CAD build for the part. Positions are in the model's coordinates, mm. Face numbers are marked on the shaded views. A direction names the side the tool comes from. Round coordinates to 2 decimals unless told otherwise and drop trailing zeros. Write each loop counter-clockwise with the first axis right and the second up, starting at its lowest first coordinate (ties: lowest second). Pieces come first, ordered by that corner, then holes. Notation, with made-up numbers: (-33, 75.5) - (0, 75.5) arc R21 ccw to (0, 107.5) - close; hole circle Ø1 at (-2, -34). An arc over 180 degrees is marked (long way). Put each result on its own line as item: value. Start each with the question number.
Item 1: Mould opens along Z. For the marked faces 4, 5, 6 and 7 say: released by +Z, released by -Z, zero draft, split by the parting line, or undercut.
Item 2: Drill centre lines: line 1 (Z direction, x = 93.25, y = 2); line 2 (X direction, y = 2, z = 2); line 3 (Z direction, x = 91.75, y = 6.75). Where is each one in solid material? Low to high. Write a range as from..to.
Item 3: Pin check, flat tips, straight feed: pin 1 Ø5 at (x, z) = (89, 29) entering from +Y; pin 2 Ø8 at (x, z) = (91, 32.5) entering from -Y. Stop position of each tip, or through.
Item 4: Cut at C-C (y = 9.5). Give the cut face in (x, z).
Item 5: 3-axis set-ups, long thin cutter, end or side, ignore diameter. For the marked faces 1, 2 and 3: which of +Z, -Z, +X, -X, +Y, -Y reach the whole face in a straight line?
Item 6: Cut at D-D (z = 34). Give the cut face in (x, y).
Item 7: Cut at A-A (z = 70.5). Give the cut face in (x, y).
Item 8: Cut at B-B (x = 88.5). Give the cut face in (y, z), and give its area (3 significant figures).
Autodesk Fusion 360 part; units mm, degrees
sketch "Sketch1" plane through (0, 0, 0) normal (0, 1, 0) x (1, 0, 0)
  line L0 (0, 0) -> (20.4, 0) construction
  line L1 (20.4, 0) -> (20.4, -88.85) construction
  line L2 (0, 0) -> (20.4, 0)
  line L3 (20.4, 0) -> (20.4, -88.85)
  line L4 (20.4, -88.85) -> (0, -88.85)
  line L5 (0, -88.85) -> (0, 0)
  line L6 (20.4, 0) -> (17.9, 0) construction
  line L7 (17.9, 0) -> (17.9, -2.5) construction
  line L8 (17.9, -2.5) -> (20.4, -2.5) construction
  line L9 (20.4, -2.5) -> (20.4, 0) construction
  circle A0 centre (17.9, -2.5) radius 1.5
  line L10 (0, 0) -> (2.5, 0) construction
  line L11 (2.5, 0) -> (2.5, -2.5) construction
  line L12 (2.5, -2.5) -> (0, -2.5) construction
  line L13 (0, -2.5) -> (0, 0) construction
  line L14 (0, -88.85) -> (2.5, -88.85) construction
  line L15 (2.5, -88.85) -> (2.5, -86.35) construction
  line L16 (2.5, -86.35) -> (0, -86.35) construction
  line L17 (0, -86.35) -> (0, -88.85) construction
  line L18 (20.4, -88.85) -> (17.9, -88.85) construction
  line L19 (17.9, -88.85) -> (17.9, -86.35) construction
  line L20 (17.9, -86.35) -> (20.4, -86.35) construction
  line L21 (20.4, -86.35) -> (20.4, -88.85) construction
  circle A1 centre (2.5, -86.35) radius 1.5
  circle A2 centre (17.9, -86.35) radius 1.5
  circle A3 centre (2.5, -2.5) radius 1.5
  circle A4 centre (2.5, -2.5) radius 2
  circle A5 centre (17.9, -2.5) radius 2
  circle A6 centre (2.5, -86.35) radius 2
  circle A7 centre (17.9, -86.35) radius 2
  dimension "d1" = 20.4
  dimension "d2" = 88.85
  dimension "d3" = 2.5
  dimension "d4" = 2.5
  dimension "d5" = 3
  dimension "d6" = 2.5
  dimension "d7" = 2.5
  dimension "d8" = 2.5
  dimension "d9" = 2.5
  dimension "d10" = 2.5
  dimension "d11" = 2.5
  dimension "d12" = 3
  dimension "d13" = 3
  dimension "d14" = 3
  dimension "d15" = 4
  dimension "d16" = 4
  dimension "d17" = 4
  dimension "d18" = 4
extrude "Extrude1" add sketch "Sketch1" along normal blind 1 contours L2 L3 L4 L5 makes body 1
extrude "Extrude2" add sketch "Sketch1" along normal blind 1 contours A0 | A1 | A2 | A3 | A4 | A5 | A6 | A7 bodies 1
extrude "Extrude3" add sketch "Sketch1" along normal blind 10 contours A4 | A5 | A6 | A7 bodies 1
extrude "Extrude4" add 4 faces at (17.7887, 1, 3.5508) (2.9404, 1, 2.5827) (17.4222, 1, 86.4974) (2.3887, 1, 87.4008) along direction (0, 1, 0) blind 5 on bodies 1 bodies 1
sketch "Sketch2" plane through (0, 0, 0) normal (0, 1, 0) x (1, 0, 0)
  line L0 (55, 0) -> (64.5, 0) construction
  line L1 (55, 0) -> (55, -75.2) construction
  line L2 (55, -75.2) -> (64.5, -75.2)
  line L3 (64.5, -75.2) -> (64.5, 0)
  line L4 (64.5, 0) -> (55, 0)
  line L5 (55, 0) -> (55, -75.2)
  line L6 (64.5, -75.2) -> (68.5, -75.2) construction
  line L7 (68.5, -75.2) -> (68.5, -79.2) construction
  line L8 (68.5, -79.2) -> (64.5, -79.2) construction
  line L9 (64.5, -79.2) -> (64.5, -75.2) construction
  line L10 (55, 0) -> (51, 0) construction
  line L11 (51, 0) -> (51, 4) construction
  line L12 (51, 4) -> (55, 4) construction
  line L13 (55, 4) -> (55, 0) construction
  line L14 (51, 4) -> (68.5, 4)
  line L15 (68.5, 4) -> (68.5, -79.2)
  line L16 (68.5, -79.2) -> (51, -79.2)
  line L17 (51, -79.2) -> (51, 4)
  line L18 (59.75, -75.2) -> (59.75, -61.2) construction
  line L19 (59.75, 0) -> (59.75, -14) construction
  line L20 (59.75, -14) -> (55, -14) construction
  line L21 (59.75, -61.2) -> (64.5, -61.2) construction
  line L22 (55, -14) -> (64.5, -14)
  line L23 (64.5, -14) -> (64.5, -61.2)
  line L24 (64.5, -61.2) -> (55, -61.2)
  line L25 (55, -61.2) -> (55, -14)
  line L26 (55, -75.2) -> (64.5, -75.2)
  line L27 (64.5, -75.2) -> (64.5, -79.2)
  line L28 (64.5, -79.2) -> (55, -79.2)
  line L29 (55, -79.2) -> (55, -75.2)
  line L30 (55, 0) -> (64.5, 0)
  line L31 (64.5, 0) -> (64.5, 4)
  line L32 (64.5, 4) -> (55, 4)
  line L33 (55, 4) -> (55, 0)
  dimension "d27" = 9.5
  dimension "d28" = 75.2
  dimension "d29" = 4
  dimension "d30" = 4
  dimension "d31" = 4
  dimension "d32" = 4
  dimension "d35" = 14
  dimension "d36" = 14
extrude "Extrude5" add sketch "Sketch2" along normal blind 1 separate body makes body 2
extrude "Extrude6" add sketch "Sketch2" along normal blind 10 contours L3 L5 L22 L23 L24 L25 bodies 2
extrude "Extrude7" add sketch "Sketch2" along normal blind 20 contours L5 L14 L16 L17 L25 L29 L33 | L3 L14 L15 L16 L23 L27 L31 bodies 2
sketch "Sketch3" plane through (0, 0, 0) normal (0, 1, 0) x (1, 0, 0)
  line L0 (85, -15) -> (94.5, -15)
  line L1 (94.5, -15) -> (94.5, -62.2)
  line L2 (94.5, -62.2) -> (85, -62.2)
  line L3 (85, -62.2) -> (85, -15)
  line L4 (94.5, -15) -> (96.5, -15)
  line L5 (96.5, -15) -> (96.5, -62.2)
  line L6 (96.5, -62.2) -> (94.5, -62.2)
  line L7 (94.5, -62.2) -> (94.5, -15)
  line L8 (85, -15) -> (83, -15)
  line L9 (83, -15) -> (83, -62.2)
  line L10 (83, -62.2) -> (85, -62.2)
  line L11 (85, -62.2) -> (85, -15)
  line L12 (85, -38.6) -> (85, -0.9) construction
  line L13 (94.5, -38.6) -> (94.5, -0.9) construction
  line L14 (85, -38.6) -> (85, -76.3) construction
  line L15 (94.5, -38.6) -> (94.5, -76.3) construction
  line L16 (83, -62.2) -> (85, -62.2)
  line L17 (85, -62.2) -> (85, -76.3)
  line L18 (85, -76.3) -> (83, -76.3)
  line L19 (83, -76.3) -> (83, -62.2)
  line L20 (94.5, -76.3) -> (96.5, -76.3)
  line L21 (96.5, -76.3) -> (96.5, -62.2)
  line L22 (96.5, -62.2) -> (94.5, -62.2)
  line L23 (94.5, -62.2) -> (94.5, -76.3)
  line L24 (83, -76.3) -> (96.5, -76.3)
  line L25 (96.5, -76.3) -> (96.5, -78.3)
  line L26 (96.5, -78.3) -> (83, -78.3)
  line L27 (83, -78.3) -> (83, -76.3)
  line L28 (85, -0.9) -> (83, -0.9)
  line L29 (83, -0.9) -> (83, -15)
  line L30 (83, -15) -> (85, -15)
  line L31 (85, -15) -> (85, -0.9)
  line L32 (94.5, -0.9) -> (96.5, -0.9)
  line L33 (96.5, -0.9) -> (96.5, -15)
  line L34 (96.5, -15) -> (94.5, -15)
  line L35 (94.5, -15) -> (94.5, -0.9)
  line L36 (96.5, -0.9) -> (83, -0.9)
  line L37 (83, -0.9) -> (83, 1.1)
  line L38 (83, 1.1) -> (96.5, 1.1)
  line L39 (96.5, 1.1) -> (96.5, -0.9)
  dimension "d41" = 9.5
  dimension "d42" = 47.2
  dimension "d43" = 2
  dimension "d44" = 2
  dimension "d49" = 37.7
  dimension "d50" = 37.7
  dimension "d51" = 37.7
  dimension "d52" = 37.7
  dimension "d53" = 2
  dimension "d54" = 2
extrude "Extrude8" add sketch "Sketch3" along normal blind 3 separate body contours L0 L1 L2 L3 L7 L11 makes body 3
extrude "Extrude9" add sketch "Sketch3" along normal blind 11 contours L3 L8 L9 L10 L11 L16 L30 | L1 L4 L5 L6 L7 L22 L34 bodies 3
extrude "Extrude10" add sketch "Sketch3" along normal blind 11 contours L8 L28 L29 L30 L31 L36 | L4 L32 L33 L34 L35 L36 | L10 L16 L17 L18 L19 L24 | L28 L32 L36 L37 L38 L39 | L6 L20 L21 L22 L23 L24 | L18 L20 L24 L25 L26 L27 bodies 3
hidden bodies 1 2
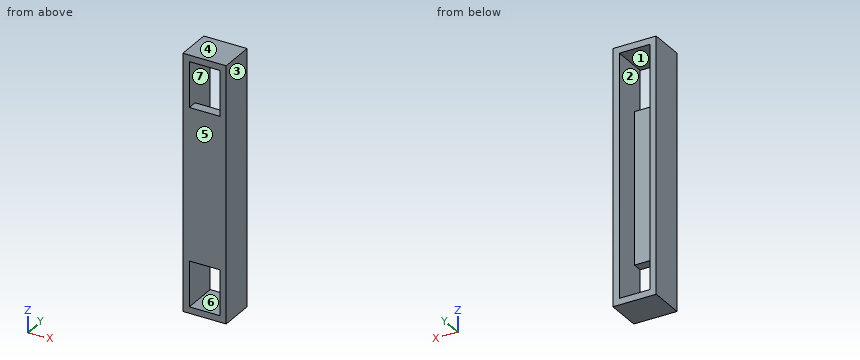
Output values:
1. face 4: released by +Z
1. face 5: zero draft
1. face 6: undercut
1. face 7: undercut
2. line 1: -1.1..0.9, 15..62.2, 76.3..78.3
2. line 2: 83..85, 94.5..96.5
2. line 3: -1.1..0.9, 76.3..78.3
3. pin 1: y = 3
3. pin 2: y = 0
4. outline: (83, -1.1) - (96.5, -1.1) - (96.5, 78.3) - (83, 78.3) - close; hole (85, 0.9) - (94.5, 0.9) - (94.5, 76.3) - (85, 76.3) - close
5. face 1: +Y, -Y
5. face 2: +Y
5. face 3: +Z, -Z, +X, +Y, -Y
6. outline: (83, 0) - (96.5, 0) - (96.5, 11) - (94.5, 11) - (94.5, 3) - (85, 3) - (85, 11) - (83, 11) - close
7. outline: (83, 0) - (85, 0) - (85, 11) - (83, 11) - close; (94.5, 0) - (96.5, 0) - (96.5, 11) - (94.5, 11) - close
8. outline: (0, -1.1) - (11, -1.1) - (11, 0.9) - (0, 0.9) - close; (0, 15) - (3, 15) - (3, 62.2) - (0, 62.2) - close; (0, 76.3) - (11, 76.3) - (11, 78.3) - (0, 78.3) - close
8. area: 186 mm2
